Could you check a few things on this model? Use its own coordinates, in mm. Face numbers are marked on the shaded views. A direction names the side the tool comes from. Coordinates: 2 decimals unless noted, no trailing zeros. Order: outer loops, then holes, each group sorted by start corner. A loop starts at its lowest first (then second) coordinate and runs counter-clockwise, first axis right, second up. Notation, with made-up numbers: (-31, -3.5) - (20, -3.5) arc R10 ccw to (20, 0.5) - close; hole circle Ø11 at (-37, -9.75). An arc over 180 degrees is marked (long way). Answer as a JSON object with one key per item and string values. Group by question number.
(1) Imagine slicing it at A-A, the plane x = -2.25. Write out the boundary of the cut face in (y, z).
(2) Imagine slicing it at C-C, the plane z = 1.85. Write out the boundary of the cut face in (x, y).
(3) Which directions (+Z, -Z, +X, -X, +Y, -Y) give clear straight access to the entire face, cutting with the end or side of a thin tool? Please do the marked faces 5 and 6.
(4) Imagine slicing it at B-B, the plane y = 2. Write out the boundary of the cut face in (x, z), and give its area (3 significant figures).
(5) Please list where these lines run through material, in increasing order: probe 1 along X at (y, z) = (1.25, 2.45); probe 2 along X at (y, z) = (2.25, 0.6); probe 3 along X at (y, z) = (0.75, 2.2).
(6) Will these pins go through, and if not, where does the flat tip stop? P1, Ø1, axis at y = 0, z = 1.5, coming from the -X side; P2, Ø2, axis at x = -4.5, y = 2.5, coming from the +Z side; P3, Ø6.5, axis at x = -6, y = -0.5, coming from the +Z side; P4, Ø3.5, axis at x = -2.32, y = 2.32, coming from the -Z side.
(7) We'd pull the mould along X, two halves only. Please class the marked faces 1, 2, 3 and 4: pulls with the +X half, pulls with the -X half, needs draft (parallel to the pull), parting line crosses it, or undercut.
(8) Imagine slicing it at D-D, the plane x = -11. Write out the boundary of the cut face in (y, z).
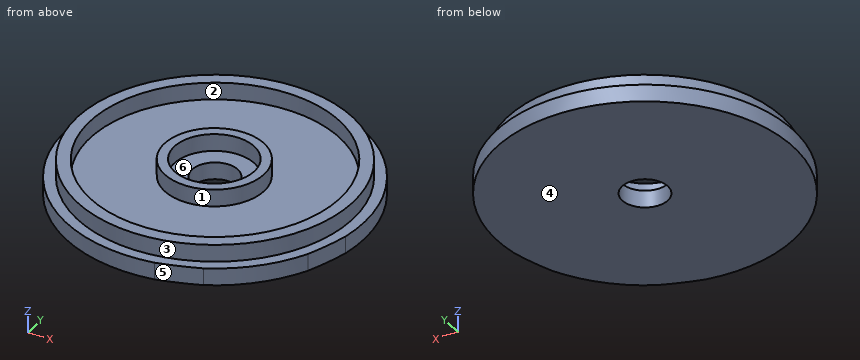
from build123d import *

# Parameters (mm, degrees)
F0_R     = 12.0291917003
F0_R_2   = 10.9089247003
F0_R_3   = 10
F0_R_4   = 4.355405347
F0_R_5   = 3.5
F0_R_6   = 2
F1_DEPTH = 1.5
F2_DEPTH = 3
F3_DEPTH = 25.4


with BuildPart() as f1:
    # F0 (on Top) → F1 (new body)
    with BuildSketch(Plane.XY):
        with BuildLine():
            ThreePointArc((9.2903810009, -3.5340649529), (9.956324904, -1.7586338449), (10.4848555288, 0.062435149))
            ThreePointArc((10.4848555288, 0.062435149), (-11.5103310146, 11.5102886119), (-0.0624775516, -10.4848979314))
            ThreePointArc((-0.0624775516, -10.4848979314), (1.7563351899, -9.9492852383), (3.5341859381, -9.2903410352))
            ThreePointArc((3.5341859381, -9.2903410352), (6.8744732182, -6.8743862374), (9.2903810009, -3.5340649529))
        make_face()
        with Locations((-2.3179612439, 2.3179188413)):
            Circle(F0_R, mode=Mode.SUBTRACT)
        with Locations((-2.3179612439, 2.3179188413)):
            Circle(F0_R)
        with Locations((-2.3179612439, 2.3179188413)):
            Circle(F0_R_2, mode=Mode.SUBTRACT)
        with Locations((-2.3179612439, 2.3179188413)):
            Circle(F0_R_2)
        with Locations((-2.4294834584, 2.4055044632)):
            Circle(F0_R_3, mode=Mode.SUBTRACT)
        with Locations((-2.4294834584, 2.4055044632)):
            Circle(F0_R_3)
        with Locations((-2.4294834584, 2.4055044632)):
            Circle(F0_R_4, mode=Mode.SUBTRACT)
        with Locations((-2.4294834584, 2.4055044632)):
            Circle(F0_R_4)
        with Locations((-2.4294834584, 2.4055044632)):
            Circle(F0_R_5, mode=Mode.SUBTRACT)
        with Locations((-2.4294834584, 2.4055044632)):
            Circle(F0_R_5)
        with Locations((-2.3179612439, 2.3179188413)):
            Circle(F0_R_6, mode=Mode.SUBTRACT)
        with Locations((-2.3179612439, 2.3179188413)):
            Circle(F0_R_6)
    extrude(amount=F1_DEPTH)

    # F0 (on Top) → F2 (join)
    with BuildSketch(Plane.XY):
        with Locations((-2.3179612439, 2.3179188413)):
            Circle(F0_R)
        with Locations((-2.3179612439, 2.3179188413)):
            Circle(F0_R_2, mode=Mode.SUBTRACT)
        with Locations((-2.4294834584, 2.4055044632)):
            Circle(F0_R_4)
        with Locations((-2.4294834584, 2.4055044632)):
            Circle(F0_R_5, mode=Mode.SUBTRACT)
    extrude(amount=F2_DEPTH)

    # F0 (on Top) → F3 (cut)
    with BuildSketch(Plane.XY):
        with Locations((-2.3179612439, 2.3179188413)):
            Circle(F0_R_6)
    extrude(amount=F3_DEPTH, mode=Mode.SUBTRACT)


solid = f1.part
Result set:
{
 "1": {"outline": "(-10.68, 0) - (0.32, 0) - (0.32, 1.5) - (-1.09, 1.5) - (-1.09, 3) - (-1.95, 3) - (-1.95, 1.5) - (-8.59, 1.5) - (-8.59, 3) - (-9.71, 3) - (-9.71, 1.5) - (-10.68, 1.5) - close; (4.32, 0) - (15.32, 0) - (15.32, 1.5) - (14.35, 1.5) - (14.35, 3) - (13.23, 3) - (13.23, 1.5) - (6.76, 1.5) - (6.76, 3) - (5.9, 3) - (5.9, 1.5) - (4.32, 1.5) - close"},
 "2": {"outline": "circle Ø24.06 at (-2.32, 2.32); circle Ø8.71 at (-2.43, 2.41); hole circle Ø21.82 at (-2.32, 2.32); hole circle Ø7 at (-2.43, 2.41)"},
 "3": {"face 5": "+Z, -Z, +X, -Y", "face 6": "+Z"},
 "4": {"outline": "(-15.31, 0) - (-4.29, 0) - (-4.29, 1.5) - (-5.91, 1.5) - (-5.91, 3) - (-6.77, 3) - (-6.77, 1.5) - (-13.22, 1.5) - (-13.22, 3) - (-14.34, 3) - (-14.34, 1.5) - (-15.31, 1.5) - close; (-0.34, 0) - (10.68, 0) - (10.68, 1.5) - (9.71, 1.5) - (9.71, 3) - (8.59, 3) - (8.59, 1.5) - (1.91, 1.5) - (1.91, 3) - (1.05, 3) - (1.05, 1.5) - (-0.34, 1.5) - close", "area": "39.0 mm^2"},
 "5": {"probe 1": "x = -14.3 to -13.17, -6.63 to -5.73, 0.87 to 1.77, 8.54 to 9.66", "probe 2": "x = -15.32 to -4.32, -0.32 to 10.68", "probe 3": "x = -14.24 to -13.11, -6.46 to -5.51, 0.65 to 1.6, 8.48 to 9.61"},
 "6": {"P1": "stops at x = -15.19", "P2": "stops at z = 1.5", "P3": "stops at z = 3", "P4": "passes through"},
 "7": {"face 1": "undercut", "face 2": "undercut", "face 3": "parting line crosses it", "face 4": "needs draft"},
 "8": {"outline": "(-7.36, 0) - (11.99, 0) - (11.99, 1.5) - (10.64, 1.5) - (10.64, 3) - (8.92, 3) - (8.92, 1.5) - (-4.29, 1.5) - (-4.29, 3) - (-6.01, 3) - (-6.01, 1.5) - (-7.36, 1.5) - close"}
}
